from build123d import *

# Parameters (mm, degrees)
F1_DEPTH = 38.1


with BuildPart() as f1:
    # F0 (on Top) → F1 (new body, symmetric)
    with BuildSketch(Plane.XY):
        with BuildLine():
            Line((31.75, -6.35), (31.75, -4.7625))
            Line((31.75, -4.7625), (0, -4.7625))
            ThreePointArc((0, -4.7625), (-1.882543, 4.374636), (3.458453, -3.274219))
            Line((3.458453, -3.274219), (4.611271, -4.365625))
            ThreePointArc((4.611271, -4.365625), (-2.510058, 5.832847), (0, -6.35))
            Line((0, -6.35), (31.75, -6.35))
        make_face()
    extrude(amount=F1_DEPTH, both=True)


solid = f1.part
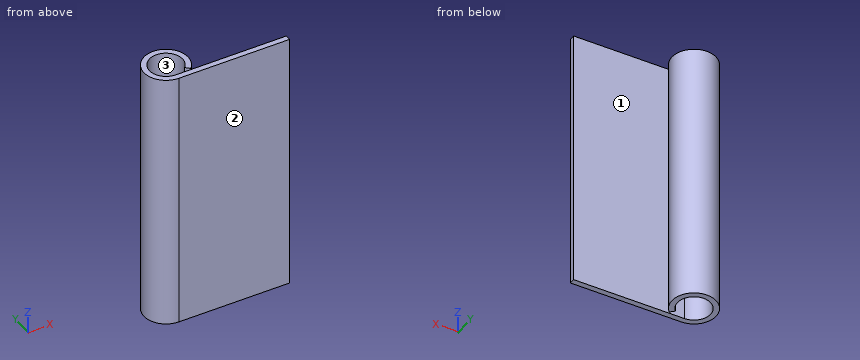
The model under review builds one solid part; all positions refer to its coordinate system, in mm. Face numbers are marked on the shaded views. Round coordinates to 2 decimals unless told otherwise and drop trailing zeros. Write each loop counter-clockwise with the first axis right and the second up, starting at its lowest first coordinate (ties: lowest second). Pieces come first, ordered by that corner, then holes. Notation, with made-up numbers: M -24.5,38 L 11.5,38 A14 cw 11.5,44 Z; hole C 12.25,-16 d11. An arc over 180 degrees is marked long. Use a Markdown table: item, result. Add a question column.
Q1. We need section C-C, the plane y = 3.5. State the section outline as (x, z) points, plus the area to 3 significant figures.
Q2. Insertion check: pin 1 (1 mm diameter, centred on y = 5, z = -24.5, fed in from -X). The pin has a flat end and moves straight along its axis. Give the tip position at first contact, or say it passes through.
Q3. To check wall thickness, follow line 1 (Y direction, x = 0, z = -7); line 2 (Y direction, x = 10.5, z = -25). State the ranges of each line that lie inside material, in increasing order.
Q4. We need section D-D, the plane x = 27. State the section outline as (y, z) points, plus the area to 3 significant figures.
Q5. We need section A-A, the plane y = 0. State the section outline as (x, z) points, plus the area to 3 significant figures.
Q6. The part is to be moulded in two halves that separate along Y. For the marked faces 1, 2 and 3, say which applies: pulls with the +Y half, pulls with the -Y half, needs draft (parallel to the pull), parting line crosses it, or undercut.
Findings below:
| question | item | result |
|---|---|---|
| 1 | outline | M -5.3,-38.1 L -3.23,-38.1 L -3.23,38.1 L -5.3,38.1 Z; M 3.23,-38.1 L 5.3,-38.1 L 5.3,38.1 L 3.23,38.1 Z |
| 1 | area | 315 mm² |
| 2 | pin 1 | stops at x = -4.48 |
| 3 | line 1 | y = -6.35 to -4.76, 4.76 to 6.35 |
| 3 | line 2 | y = -6.35 to -4.76 |
| 4 | outline | M -6.35,-38.1 L -4.76,-38.1 L -4.76,38.1 L -6.35,38.1 Z |
| 4 | area | 121 mm² |
| 5 | outline | M -6.35,-38.1 L -4.76,-38.1 L -4.76,38.1 L -6.35,38.1 Z; M 4.76,-38.1 L 6.35,-38.1 L 6.35,38.1 L 4.76,38.1 Z |
| 5 | area | 242 mm² |
| 6 | face 1 | undercut |
| 6 | face 2 | pulls with the -Y half |
| 6 | face 3 | undercut |
